from build123d import *

# Parameters (mm, degrees)
SKETCH1_R           = 2.4
BOSS_EXTRUDE1_DEPTH = 3
SKETCH2_W           = 8
SKETCH2_H           = 8
BOSS_EXTRUDE2_DEPTH = 25
SKETCH3_R           = 2.5
CUT_EXTRUDE1_DEPTH  = 4
FILLET1_R           = 1


with BuildPart() as part:
    # Sketch1 → Boss-Extrude1 (new body)
    with BuildSketch(Plane(origin=(0, 0, 0), x_dir=(1, 0, 0), z_dir=(0, 1, 0))):
        with Locations(Location((0, 0, 0), (0, 0, 270))):
            Circle(SKETCH1_R)
    extrude(amount=BOSS_EXTRUDE1_DEPTH)

    # Sketch2 → Boss-Extrude2 (add)
    with BuildSketch(Plane(origin=(0, 3, 0), x_dir=(1, 0, 0), z_dir=(0, 1, 0))):
        Rectangle(SKETCH2_W, SKETCH2_H)
    extrude(amount=BOSS_EXTRUDE2_DEPTH)

    # Sketch3 → Cut-Extrude1 (cut)
    with BuildSketch(Plane(origin=(0, 28, 0), x_dir=(1, 0, 0), z_dir=(0, 1, 0))):
        with Locations(Location((0, 0, 0), (0, 0, 270))):
            Circle(SKETCH3_R)
    extrude(amount=-CUT_EXTRUDE1_DEPTH, mode=Mode.SUBTRACT)

    # Fillet1
    fillet1_edges = [part.edges().sort_by_distance(p)[0] for p in [
        (4, 15.5, 4),
        (4, 15.5, -4),
        (-4, 15.5, -4),
        (-4, 15.5, 4),
    ]]
    fillet(fillet1_edges, radius=FILLET1_R)


solid = part.part
CAD build for the part. Positions are in the model's coordinates, mm. A direction names the side the tool comes from. Round coordinates to 2 decimals unless told otherwise and drop trailing zeros. Order: outer loops, then holes, each group sorted by start corner. A loop starts at its lowest first (then second) coordinate and runs counter-clockwise, first axis right, second up. Notation, with made-up numbers: (15.25, 8) -> (41.25, 8) arc R16 ccw to (41.25, 14) -> close; hole circle Ø4 at (-34, 63). An arc over 180 degrees is marked (long way). Write each question's results on one line, items separated by ' | '.
1. Wall check: line 1 along X through (y, z) = (25.25, 0); line 2 along Y through (x, z) = (3.25, -0.5); line 3 along Z through (x, y) = (-1.75, 25). Give the ranges that are in metal, low to high. Write a range as [from, to].
Findings below:
line 1: x = [-4, -2.5], [2.5, 4] | line 2: y = [3, 28] | line 3: z = [-4, -1.79], [1.79, 4]
2. Pull direction X, two halves, no side cores. Call faces 1 (the face through (4, 15, 0)), 2 (the face through (0, 15, 4)), 3 (the face through (0, 24, 0)): pulls with the +X half, pulls with the -X half, needs draft (parallel to the pull), parting line crosses it, or undercut.
Findings below:
face 1: pulls with the +X half | face 2: needs draft | face 3: undercut
3. 3-axis set-ups, long thin cutter, end or side, ignore diameter. For faces 4 (the face through (0, 15, -4)), 5 (the face through (-2, 3, 2)), 6 (the face through (-2.44, 26.03, -0.54)): which of +Z, -Z, +X, -X, +Y, -Y reach the whole face in a straight line?
Findings below:
face 4: -Z, +X, -X, +Y, -Y | face 5: -Y | face 6: +Y
4. Cut at C-C (z = 0). Give the cut face in (x, y), plus the area to 3 significant figures.
Findings below:
outline: (-4, 3) -> (-2.4, 3) -> (-2.4, 0) -> (2.4, 0) -> (2.4, 3) -> (4, 3) -> (4, 28) -> (2.5, 28) -> (2.5, 24) -> (-2.5, 24) -> (-2.5, 28) -> (-4, 28) -> close | area: 194 mm²
5. Cut at A-A (x = 0). Give the cut face in (y, z), plus the area to 3 significant figures.
Findings below:
outline: (0, -2.4) -> (3, -2.4) -> (3, -4) -> (28, -4) -> (28, -2.5) -> (24, -2.5) -> (24, 2.5) -> (28, 2.5) -> (28, 4) -> (3, 4) -> (3, 2.4) -> (0, 2.4) -> close | area: 194 mm²
6. Cut at B-B (y = 24.75). Give the cut face in (x, z).
Findings below:
outline: (-4, -3) arc R1 ccw to (-3, -4) -> (3, -4) arc R1 ccw to (4, -3) -> (4, 3) arc R1 ccw to (3, 4) -> (-3, 4) arc R1 ccw to (-4, 3) -> close; hole circle Ø5 at (0, 0)
7. Flat gauge pin, fed straight in: P1, Ø1.5, axis at x = -1, z = -0.5, coming from the +Y side. Where does the tip first touch, or does it go through?
Findings below:
P1: stops at y = 24
